Part model, mm, in its own coordinate system. A direction names the side the tool comes from. Give positions to 0.01 mm unless a question says otherwise; leave off trailing zeros. Write each loop counter-clockwise with the first axis right and the second up, starting at its lowest first coordinate (ties: lowest second). Pieces come first, ordered by that corner, then holes.
```python
from build123d import *

# Parameters (mm, degrees)
SKETCH1_R           = 1.4
BOSS_EXTRUDE1_DEPTH = 8
CUT_EXTRUDE1_DEPTH  = 2


with BuildPart() as part:
    # Sketch1 → Boss-Extrude1 (new body)
    with BuildSketch(Plane(origin=(0, 0, 0), x_dir=(1, 0, 0), z_dir=(0, 1, 0))):
        with BuildLine():
            Line((-15, 36), (-15, -40))
            ThreePointArc((-15, -40), (-13.535533906, -43.535533906), (-10, -45))
            Line((-10, -45), (25, -45))
            ThreePointArc((25, -45), (28.535533906, -43.535533906), (30, -40))
            Line((30, -40), (30, 36))
            ThreePointArc((30, 36), (28.535533906, 39.535533906), (25, 41))
            Line((25, 41), (-10, 41))
            ThreePointArc((-10, 41), (-13.535533906, 39.535533906), (-15, 36))
        make_face()
        with Locations(Location((18.5, -20, 0), (0, 0, 270))):
            Circle(SKETCH1_R, mode=Mode.SUBTRACT)
        with Locations(Location((-3.5, -20, 0), (0, 0, 270))):
            Circle(SKETCH1_R, mode=Mode.SUBTRACT)
        with Locations(Location((18.5, 27, 0), (0, 0, 270))):
            Circle(SKETCH1_R, mode=Mode.SUBTRACT)
        with Locations(Location((-3.5, 27, 0), (0, 0, 270))):
            Circle(SKETCH1_R, mode=Mode.SUBTRACT)
        with BuildLine():
            Line((-2.2, -37.8), (0.4, -37.8))
            ThreePointArc((0.4, -37.8), (2, -39.4), (3.6, -37.8))
            Line((3.6, -37.8), (3.6, -30))
            ThreePointArc((3.6, -30), (2, -28.4), (0.4, -30))
            Line((0.4, -30), (-2.2, -30))
            ThreePointArc((-2.2, -30), (-3.8, -28.4), (-5.4, -30))
            Line((-5.4, -30), (-5.4, -37.8))
            ThreePointArc((-5.4, -37.8), (-3.8, -39.4), (-2.2, -37.8))
        make_face(mode=Mode.SUBTRACT)
        with BuildLine():
            Line((14.6, -37.8), (17.2, -37.8))
            ThreePointArc((17.2, -37.8), (18.8, -39.4), (20.4, -37.8))
            Line((20.4, -37.8), (20.4, -30))
            ThreePointArc((20.4, -30), (18.8, -28.4), (17.2, -30))
            Line((17.2, -30), (14.6, -30))
            ThreePointArc((14.6, -30), (13, -28.4), (11.4, -30))
            Line((11.4, -30), (11.4, -37.8))
            ThreePointArc((11.4, -37.8), (13, -39.4), (14.6, -37.8))
        make_face(mode=Mode.SUBTRACT)
        with BuildLine():
            Line((18.5, -16), (22.5, -16))
            Line((22.5, -16), (22.5, 23))
            Line((22.5, 23), (18.5, 23))
            ThreePointArc((18.5, 23), (15.671572875, 24.171572875), (14.5, 27))
            Line((14.5, 27), (14.5, 31))
            Line((14.5, 31), (0.5, 31))
            Line((0.5, 31), (0.5, 27))
            ThreePointArc((0.5, 27), (-0.671572875, 24.171572875), (-3.5, 23))
            Line((-3.5, 23), (-7.5, 23))
            Line((-7.5, 23), (-7.5, -16))
            Line((-7.5, -16), (-3.5, -16))
            ThreePointArc((-3.5, -16), (-0.671572875, -17.171572875), (0.5, -20))
            Line((0.5, -20), (0.5, -24))
            Line((0.5, -24), (14.5, -24))
            Line((14.5, -24), (14.5, -20))
            ThreePointArc((14.5, -20), (15.671572875, -17.171572875), (18.5, -16))
        make_face(mode=Mode.SUBTRACT)
    extrude(amount=BOSS_EXTRUDE1_DEPTH)

    # Sketch2 → Cut-Extrude1 (cut)
    with BuildSketch(Plane(origin=(0, 8, 0), x_dir=(1, 0, 0), z_dir=(0, 1, 0))):
        with BuildLine():
            Line((-4.3, 31), (19.3, 31))
            ThreePointArc((19.3, 31), (21.5627417, 30.0627417), (22.5, 27.8))
            Line((22.5, 27.8), (22.5, -20.8))
            ThreePointArc((22.5, -20.8), (21.5627417, -23.0627417), (19.3, -24))
            Line((19.3, -24), (-4.3, -24))
            ThreePointArc((-4.3, -24), (-6.5627417, -23.0627417), (-7.5, -20.8))
            Line((-7.5, -20.8), (-7.5, 27.8))
            ThreePointArc((-7.5, 27.8), (-6.5627417, 30.0627417), (-4.3, 31))
        make_face()
    extrude(amount=-CUT_EXTRUDE1_DEPTH, mode=Mode.SUBTRACT)


solid = part.part
```
1) Pin check, flat tip, straight feed: pin 1 Ø12 at (x, z) = (21.5, -9.5) entering from -Y. Stop position of the tip, or through.
Answers follow:
pin 1: stops at y = 0
2) Wall check: L1, parallel to X at y = 1, z = 37; L2, parallel to X at y = 4.35, z = -27; L3, parallel to X at y = 2.5, z = 3.5. Give the ranges that are in metal, low to high.
Answers follow:
L1: x = -15 to -5.4, 3.6 to 11.4, 20.4 to 30
L2: x = -15 to -4.9, -2.1 to 0.5, 14.5 to 17.1, 19.9 to 30
L3: x = -15 to -7.5, 22.5 to 30
3) Saw through at C-C, the plane y = 5. Count the separate pieces of the cut face and the enclosed holes in it, then the cut area to 3 significant figures.
Answers follow:
separate pieces: 1
enclosed holes: 7
area: 2,240 mm2
4) Saw through at A-A, the plane x = 2. Write the cut outline in (y, z).
Answers follow:
outline: (0, -41) - (8, -41) - (8, -31) - (0, -31) - close; (0, 24) - (8, 24) - (8, 28.4) - (0, 28.4) - close; (0, 39.4) - (8, 39.4) - (8, 45) - (0, 45) - close
5) Saw through at B-B, the plane z = -11.5. Write the cut outline in (x, y).
Answers follow:
outline: (-15, 0) - (-7.5, 0) - (-7.5, 8) - (-15, 8) - close; (22.5, 0) - (30, 0) - (30, 8) - (22.5, 8) - close
6) Two-plate mould, pull along X, no slides. Class faces 4 (the face through (7, 4, 45)), 5 (the face through (-13, 4, -40)), 6 (the face through (-3.8, 3.9, 28.4)): +X half, -X half, draft (parallel to the pull), parting line (faces both ways), or undercut.
Answers follow:
face 4: draft
face 5: -X half
face 6: undercut
7) 3-axis set-ups, long thin cutter, end or side, ignore diameter. For faces 1 (the face through (21.587, 7.014, 23.038)), 2 (the face through (-14, 4, 43)), 3 (the face through (18.8, 3.9, 28.4)): which of +Z, -Z, +X, -X, +Y, -Y reach the whole face in a straight line?
Answers follow:
face 1: +Y
face 2: +Z, -X, +Y, -Y
face 3: +Y, -Y
